```python
from build123d import *

# Parameters (mm, degrees)
SKETCH1_R           = 17
SKETCH1_R_2         = 15
BOSS_EXTRUDE1_DEPTH = 20
MOVE_FACE1_BY       = 0.15
MOVE_FACE2_BY       = 0.05


with BuildPart() as part:
    # Sketch1 → Boss-Extrude1 (new body)
    with BuildSketch(Plane.XY):
        Circle(SKETCH1_R)
        Circle(SKETCH1_R_2, mode=Mode.SUBTRACT)
    extrude(amount=BOSS_EXTRUDE1_DEPTH)

    # Move Face1: a curved face moved inward by 0.15
    add(Solid.thicken(part.faces().sort_by_distance((-17, 0, 10))[0], -MOVE_FACE1_BY), mode=Mode.SUBTRACT)

    # Move Face2: a curved face moved inward by 0.05
    add(Solid.thicken(part.faces().sort_by_distance((-15, 0, 10))[0], -MOVE_FACE2_BY), mode=Mode.SUBTRACT)


solid = part.part
```
Build history of the part. All positions in model axes, mm. Give positions to 0.01 mm unless a question says otherwise; leave off trailing zeros. Order: outer loops, then holes, each group sorted by start corner. A loop starts at its lowest first (then second) coordinate and runs counter-clockwise, first axis right, second up. Notation, with made-up numbers: M 18.5,32 L 59.5,32 A14 ccw 59.5,59 Z; hole C 70.25,5 d8. An arc over 180 degrees is marked long. Write item = value, one per line. Start each with the question number.
(1) Slice it at A-A on x = 0. Write the cut outline in (y, z).
(2) Pin check, flat tips, straight feed: pin 1 Ø4 at (y, z) = (-5.5, 4.5) entering from -X; pin 2 Ø12 at (x, z) = (9.5, 5) entering from -Y; pin 3 Ø1 at (x, z) = (-10.5, 6.5) entering from +Y. Stop position of each tip, or through.
(3) Probe L1, parallel to Y at x = 0, z = 14.5; L2, parallel to X at y = -0.5, z = 12.5; L3, parallel to X at y = 13, z = 14.5. List the from-to ranges inside material, lowest first. Write a range as [from, to].
(4) Slice it at C-C on z = 15. Write the cut outline in (x, y).
Responses:
q1.outline = M -16.85,0 L -15.05,0 L -15.05,20 L -16.85,20 Z; M 15.05,0 L 16.85,0 L 16.85,20 L 15.05,20 Z
q2.pin_1 = -16.48
q2.pin_2 = -16.48
q2.pin_3 = 13.56
q3.L1 = [-16.85, -15.05], [15.05, 16.85]
q3.L2 = [-16.84, -15.04], [15.04, 16.84]
q3.L3 = [-10.72, -7.58], [7.58, 10.72]
q4.outline = C 0,0 d33.7; hole C 0,0 d30.1
